Design review of the part shown in the three views and the two pictorial views. Dimensions are in mm from the part's minimum x, y and z. Give positions to 0.01 mm unless a question says otherwise; leave off trailing zeros. Order: outer loops, then holes, each group sorted by start corner. A loop starts at its lowest first (then second) coordinate and runs counter-clockwise, first axis right, second up. Notation, with made-up numbers: M -32.75,65.5 L 24.25,65.5 A25 cw 24.25,81.5 Z; hole C 31,26.25 d7. An arc over 180 degrees is marked long. Answer as a JSON object with one key per item and string values.
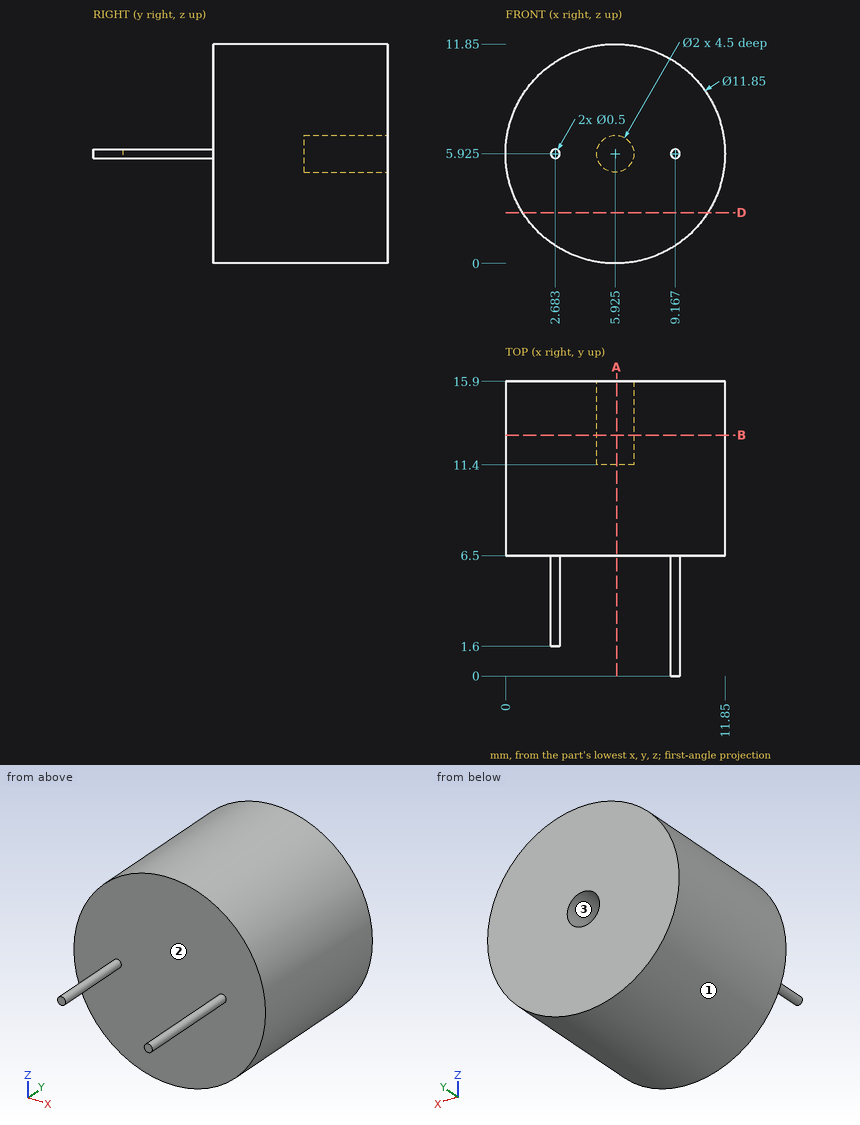
(1) We need section D-D (z = 2.75). Write out the cut boundary in (x, y).
Checked values:
{"outline": "M 0.92,6.5 L 10.93,6.5 L 10.93,15.9 L 0.92,15.9 Z"}
(2) Draft analysis for pull direction Z (two halves, no side actions). For the marked faces 1, 2 and 3, state which applies: +Z half, -Z half, draft (parallel to the pull), parting line (faces both ways), or undercut.
Checked values:
{"face 1": "parting line", "face 2": "draft", "face 3": "undercut"}
(3) Insertion check: pin 1 (3.5 mm diameter, centred on x = 3, z = 7.5, fed in from -Y); pin 2 (1.5 mm diameter, centred on y = 7, z = 2.5, fed in from +X); pin 3 (1.2 mm diameter, centred on x = 5.925, z = 5.925, fed in from +Y). Each pin has a flat end and moves straight along its axis. Give the tip position at first contact, or say it passes through.
Checked values:
{"pin 1": "stops at y = 1.6", "pin 2": "stops at x = 11.21", "pin 3": "stops at y = 11.4"}
(4) We need section A-A (x = 6). Write out the cut boundary in (y, z), plus the area to 3 significant figures.
Checked values:
{"outline": "M 6.5,0 L 15.9,0 L 15.9,4.93 L 11.4,4.93 L 11.4,6.92 L 15.9,6.92 L 15.9,11.85 L 6.5,11.85 Z", "area": "102 mm^2"}
(5) To check wall thickness, follow L1, parallel to X at y = 14, z = 6; L2, parallel to Y at x = 7.5, z = 4.5; L3, parallel to Y at x = 6, z = 5.5. State the ranges of each line that lie inside material, in increasing order. Write a range as from..to.
Checked values:
{"L1": "x = 0..4.93, 6.92..11.85", "L2": "y = 6.5..15.9", "L3": "y = 6.5..11.4"}
(6) We need section B-B (y = 13). Write out the cut boundary in (x, z) (3 decimals).
Checked values:
{"outline": "C 5.925,5.925 d11.85; hole C 5.925,5.925 d2"}
